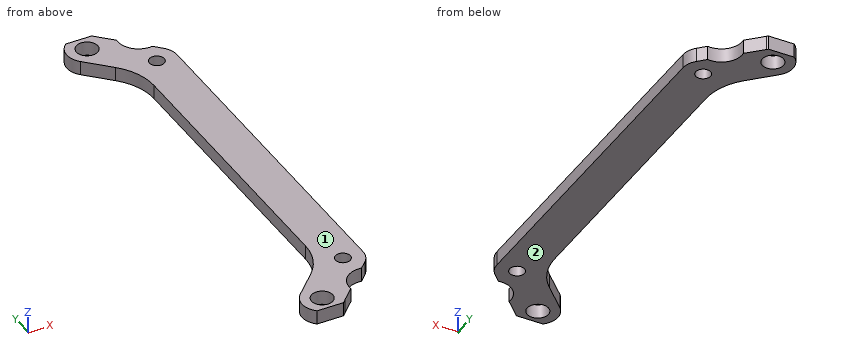
from build123d import *

# Parameters (mm, degrees)
SKIZZE1_R                       = 2.85
SKIZZE1_R_2                     = 1.05
LINEAR_AUSTRAGEN_D_NN1_DEPTH    = 2
LINEAR_AUSTRAGEN_D_NN1_2_DEPTH  = 2
LINEAR_AUSTRAGEN_D_NN1_3_DEPTH  = 2
LINEAR_AUSTRAGEN_D_NN1_4_DEPTH  = 2
AUFSATZ_LINEAR_AUSTRAGEN1_DEPTH = 2
SKIZZE4_R                       = 2.9
SCHNITT_LINEAR_AUSTRAGEN1_DEPTH = 2
SKIZZE7_R                       = 1.5
SCHNITT_LINEAR_AUSTRAGEN3_DEPTH = 4.5
VERRUNDUNG3_R                   = 8
VERRUNDUNG4_R                   = 8
SKIZZE8_W                       = 8.364298592
SKIZZE8_H                       = 2.396021337
SKIZZE8_W_2                     = 8.747208858
SKIZZE8_H_2                     = 3.084567941
SCHNITT_LINEAR_AUSTRAGEN4_DEPTH = 10


with BuildPart() as part:
    # Skizze1 → Linear-Austragen-Dünn1 (new body)
    with BuildSketch(Plane.XY):
        with Locations((43.573867598, -31.049552882)):
            Circle(SKIZZE1_R)
        with Locations((43.573867598, -31.049552882)):
            Circle(SKIZZE1_R_2, mode=Mode.SUBTRACT)
    extrude(amount=LINEAR_AUSTRAGEN_D_NN1_DEPTH)



with BuildPart() as body_2:
    # Skizze1 → Linear-Austragen-D_nn1 2 (new body)
    with BuildSketch(Plane.XY):
        with Locations((49.973867598, -24.649552882)):
            Circle(SKIZZE1_R)
        with Locations((49.973867598, -24.649552882)):
            Circle(SKIZZE1_R_2, mode=Mode.SUBTRACT)
    extrude(amount=LINEAR_AUSTRAGEN_D_NN1_2_DEPTH)


with BuildPart() as body_3:
    # Skizze1 → Linear-Austragen-D_nn1 3 (new body)
    with BuildSketch(Plane.XY):
        with Locations((49.973867598, 23.890447118)):
            Circle(SKIZZE1_R)
        with Locations((49.973867598, 23.890447118)):
            Circle(SKIZZE1_R_2, mode=Mode.SUBTRACT)
    extrude(amount=LINEAR_AUSTRAGEN_D_NN1_3_DEPTH)


with BuildPart() as body_4:
    # Skizze1 → Linear-Austragen-D_nn1 4 (new body)
    with BuildSketch(Plane.XY):
        with Locations((43.573867598, 30.290447118)):
            Circle(SKIZZE1_R)
        with Locations((43.573867598, 30.290447118)):
            Circle(SKIZZE1_R_2, mode=Mode.SUBTRACT)
    extrude(amount=LINEAR_AUSTRAGEN_D_NN1_4_DEPTH)


with BuildPart() as part_1:
    add(part.part)

    add(body_2.part)  # Aufsatz-Linear austragen1 merges body 2

    add(body_3.part)  # Aufsatz-Linear austragen1 merges body 3

    add(body_4.part)  # Aufsatz-Linear austragen1 merges body 4
    # Skizze3 → Aufsatz-Linear austragen1 (add)
    with BuildSketch(Plane(origin=(0, 0, 0), x_dir=(-1, 0, 0), z_dir=(0, 0, -1))):
        Polygon((-41.562362318, -29.03055647), (-47.123867598, -23.489686183), (-47.123867598, -24.649552882), (-48.59326597, -26.13202553), (-51.989121924, -26.664807209), (-45.264844081, -33.343697283), (-44.884208679, -29.808371771), align=None)
        with BuildLine():
            Line((-47.123867598, 22.709939373), (-47.958612175, 21.875193888))
            ThreePointArc((-47.958612175, 21.875193888), (-51.064514663, 21.257390153), (-52.823867598, 23.890447118))
            Line((-52.823867598, 23.890447118), (-52.823867598, -24.649552882))
            Line((-52.823867598, -24.649552882), (-50.178691981, -22.827758624))
            Line((-50.178691981, -22.827758624), (-47.123867598, -24.649552882))
            Line((-47.123867598, -24.649552882), (-47.123867598, -23.489686183))
            Line((-47.123867598, -23.489686183), (-47.123867598, 22.709939373))
        make_face()
        with BuildLine():
            ThreePointArc((-47.123867598, 23.890447118), (-47.340810633, 22.799800052), (-47.958612175, 21.875193888))
            Line((-47.958612175, 21.875193888), (-47.123867598, 22.709939373))
            Line((-47.123867598, 22.709939373), (-41.562362318, 28.271450706))
            Line((-41.562362318, 28.271450706), (-44.884208679, 28.654046934))
            Line((-44.884208679, 28.654046934), (-45.589121924, 32.305701444))
            Line((-45.589121924, 32.305701444), (-51.989121924, 25.905701444))
            ThreePointArc((-51.989121924, 25.905701444), (-48.883219815, 26.523503785), (-47.123867598, 23.890447118))
        make_face()
    extrude(amount=-AUFSATZ_LINEAR_AUSTRAGEN1_DEPTH)

    # Skizze4 → Schnitt-Linear austragen1 (cut)
    with BuildSketch(Plane(origin=(0, 0, 0), x_dir=(-1, 0, 0), z_dir=(0, 0, -1))):
        with Locations((-50.573867598, 29.790447118)):
            Circle(SKIZZE4_R)
        with Locations((-50.573867598, -30.549552882)):
            Circle(SKIZZE4_R)
    extrude(amount=-SCHNITT_LINEAR_AUSTRAGEN1_DEPTH, mode=Mode.SUBTRACT)

    # Skizze7 → Schnitt-Linear austragen3 (cut)
    with BuildSketch(Plane.XY.offset(2)):
        with Locations((43.573867598, -31.049552882)):
            Circle(SKIZZE7_R)
        with Locations((43.573867598, 30.290447118)):
            Circle(SKIZZE7_R)
    extrude(amount=-SCHNITT_LINEAR_AUSTRAGEN3_DEPTH, mode=Mode.SUBTRACT)

    # Verrundung3
    verrundung3_edges = [part_1.edges().sort_by_distance(p)[0] for p in [
        (47.123867598, 22.709939373, 1),
    ]]
    fillet(verrundung3_edges, radius=VERRUNDUNG3_R)

    # Verrundung4
    verrundung4_edges = [part_1.edges().sort_by_distance(p)[0] for p in [
        (47.123867598, -23.489686183, 1),
    ]]
    fillet(verrundung4_edges, radius=VERRUNDUNG4_R)

    # Skizze8 → Schnitt-Linear austragen4 (cut)
    with BuildSketch(Plane(origin=(0, 0, 0), x_dir=(-1, 0, 0), z_dir=(0, 0, -1))):
        with Locations((-42.948718638, 33.685978487)):
            Rectangle(SKIZZE8_W, SKIZZE8_H)
        with Locations((-43.64204941, -34.737574597)):
            Rectangle(SKIZZE8_W_2, SKIZZE8_H_2)
    extrude(amount=-SCHNITT_LINEAR_AUSTRAGEN4_DEPTH, mode=Mode.SUBTRACT)


solid = part_1.part
Source: CAD feature listing. Evaluate the final solid. Frame: model axes, mm. Face numbers are marked on the shaded views. Round coordinates to 2 decimals unless told otherwise and drop trailing zeros. Loops run counter-clockwise (first coordinate to the right, second up) from the corner with the lowest first, then second, coordinate; pieces in that order, holes last. Notation, with made-up numbers: (-35.5, 83) - (15.5, 83) arc R25 cw to (15.5, 120) - close; hole circle Ø8 at (26.25, 22.5). An arc over 180 degrees is marked (long way). Write item = value, one per line. Start each with the question number.
Item 1: Mould query, pull axis Z, two halves, no side actions, for the marked faces 1 and 2. Classes: released by +Z, released by -Z, zero draft, split by the parting line, or undercut.
Item 2: Section query C-C on y = 11. Output: boundary loops of the cut face in (x, z).
Item 3: Material intervals for line 1 (Y direction, x = 44.75, z = 1.65); line 2 (Y direction, x = 49.5, z = 0.65); line 3 (Y direction, x = 50.5, z = 1.8), sorted ascending.
Item 4: Section query B-B on x = 50.25. Output: boundary loops of the cut face in (y, z), plus the area to 3 significant figures.
Item 5: First-contact query: pin 1 Ø1.3 at (x, y) = (49.97, 23.89) entering from -Z; pin 2 Ø1.5 at (x, y) = (46.5, 20.5) entering from -Z; pin 3 Ø1 at (y, z) = (-6, 1) entering from -X. Flat tips, straight axial feed; report the tip coordinate or a pass-through.
Item 6: Section query D-D on y = 20.5. Output: boundary loops of the cut face in (x, z), plus the area to 3 significant figures.
Item 7: Section query A-A on z = 1.45. Output: boundary loops of the cut face in (x, y), plus the area to 3 significant figures.
Results list:
q1.face_1 = released by +Z
q1.face_2 = released by -Z
q2.outline = (47.12, 0) - (52.82, 0) - (52.82, 2) - (47.12, 2) - close
q3.line_1 = -33.2 to -31.98, -30.12 to -25.85, 25.08 to 29.36, 31.22 to 32.49
q3.line_2 = -27.86 to -25.59, -23.71 to 22.95, 24.83 to 27.1
q3.line_3 = -27.65 to -25.56, -23.74 to 22.98, 24.8 to 26.89
q4.outline = (-27.67, 0) - (-25.66, 0) - (-25.66, 2) - (-27.67, 2) - close; (-23.64, 0) - (22.88, 0) - (22.88, 2) - (-23.64, 2) - close; (24.9, 0) - (26.91, 0) - (26.91, 2) - (24.9, 2) - close
q4.area = 101 mm²
q5.pin_1 = through
q5.pin_2 = 0
q5.pin_3 = 47.12
q6.outline = (47.05, 0) - (52.82, 0) - (52.82, 2) - (47.05, 2) - close
q6.area = 11.6 mm²
q7.outline = (41.56, -29.03) arc R2.85 ccw to (41.7, -33.2) - (45.45, -33.2) arc R2.85 ccw to (45.86, -32.76) - (47.7, -30.93) arc R2.9 cw to (50.97, -27.68) - (51.98, -26.68) arc R2.85 ccw to (52.82, -24.65) - (52.82, 23.89) arc R2.85 ccw to (51.99, 25.91) - (50.98, 26.92) arc R2.9 cw to (47.7, 30.19) - (45.59, 32.31) arc R2.85 ccw to (45.39, 32.49) - (41.76, 32.49) arc R2.85 ccw to (41.56, 28.27) - (44.78, 25.05) arc R8 cw to (47.12, 19.4) - (47.12, -20.17) arc R8 cw to (44.77, -25.83) - close; hole circle Ø3 at (43.57, -31.05); hole circle Ø3 at (43.57, 30.29); hole circle Ø2.1 at (49.97, -24.65); hole circle Ø2.1 at (49.97, 23.89)
q7.area = 376 mm²
